The model under review builds one solid part; all positions refer to its coordinate system, in mm. Round coordinates to 2 decimals unless told otherwise and drop trailing zeros. Answer in a Markdown table with one row per item. Add a question column.
Autodesk Inventor part; units mm, degrees
ref_plane "YZ Plane" through (0, 0, 0) normal (1, 0, 0) x (0, 1, 0)
ref_plane "XZ Plane" through (0, 0, 0) normal (0, 1, 0) x (-1, 0, 0)
ref_plane "XY Plane" through (0, 0, 0) normal (0, 0, 1) x (1, 0, 0)
sketch "Skizze1" plane through (0, 0, 0) normal (0, 1, 0) x (-1, 0, 0)
  line L0 (0, -493.487354) -> (0, 702.145893)
  line L1 (0, -500) -> (50, -500)
  line L2 (300, 0) -> (300, -250)
  arc A0 (50, -500) -> (300, -250) centre (50, -250) ccw
  line L3 (300, 0) -> (305, 0)
  line L4 (305, 0) -> (305, -250)
  line L5 (0, -500) -> (0, -505)
  line L6 (0, -505) -> (50, -505)
  arc A1 (50, -505) -> (305, -250) centre (50, -250) ccw
  point P0 (0, 0)
  dimension "d0" = 0
  dimension "d1" = 600
  dimension "d2" = 50
  dimension "d3" = 500
  dimension "d4" = 5
  dimension "d5" = 5
  dimension "d6" = 50
revolve "Umdrehung1" add sketch "Skizze1" angle 360 about axis through (0, 0, -493.487354) along (0, 0, 1)
sketch "Skizze2" plane through (0, 0, 0) normal (0, 1, 0) x (-1, 0, 0)
  line L0 (-305, -250) -> (305, -250)
  line L1 (-50, -505) -> (50, -505)
  arc A0 (-305, -250) -> (-50, -505) centre (-50, -250) ccw
  line L2 (-101.948734, -499.652416) -> (-102.850213, -502.129245)
  line L3 (-102.850213, -502.129245) -> (-187.422693, -471.347829)
  line L4 (-187.422693, -471.347829) -> (-185.486683, -466.028607)
  point P0 (0, 0)
  point P1 (-137.214011, -489.622028)
  dimension "d8" = 90
extrude "Extrusion1" add sketch "Skizze2" along normal blind 10
sketch "Skizze3" plane through (137.214011, 0, -489.622028) normal (0.3420157, 0, -0.9396942) x (-0.9396942, 0, -0.3420157)
  line L0 (-53.430873, 0) -> (0, 0)
  circle A0 centre (0, 0) radius 105
  point P0 (-38.519221, 0)
  dimension "d12" = 210
extrude "Extrusion2" add sketch "Skizze3" against normal up to surface
sketch "Skizze4" plane through (137.214011, 0, -489.622028) normal (0.3420157, 0, -0.9396942) x (-0.9396942, 0, -0.3420157)
  circle A0 centre (0, 0) radius 100
  point P0 (-38.519221, 0)
  dimension "d15" = 200
extrude "Extrusion3" cut sketch "Skizze4" against normal through all
equation "\"d5\" = d4"
equation "\"d6\" = d2"
properties part number "Tank_3"
1. For L1, parallel to Y at x = 0, z = -96; L2, parallel to Y at x = -258, z = -113, list the stretches that pass through material, from the lowest coordinate up.
2. Insertion check: pin 1 Ø10 at (x, z) = (-156.5, -337.5) entering from +Y; pin 2 Ø8 at (x, z) = (166.5, -304.5) entering from +Y; pin 3 Ø10 at (y, z) = (165, -149) entering from +X. Each pin has a flat end and moves straight along its axis. Give the tip position at first contact, or say it passes through.
3. Mouldability with a two-part tool opening along Y and no side actions: class faces 1 (the cylindrical face through (39.054, 297.447, -126.75)), 2 (the cylindrical face through (304.705, 13.41, -126.75)), 3 (the flat face through (-5, -1, -500)), 4 (the flat face through (49.97, -38.399, -521.376)) as pulls with the +Y half, pulls with the -Y half, needs draft (parallel to the pull), parting line crosses it, or undercut.
Filled in:
| question | item | result |
|---|---|---|
| 1 | L1 | -305 to -300, 300 to 305 |
| 1 | L2 | -162.67 to -153.09, 153.09 to 162.67 |
| 2 | pin 1 | y = 247.37 |
| 2 | pin 2 | y = 251.31 |
| 2 | pin 3 | x = 259.66 |
| 3 | face 1 | undercut |
| 3 | face 2 | parting line crosses it |
| 3 | face 3 | undercut |
| 3 | face 4 | needs draft |
